from build123d import *

# Parameters (mm, degrees)
F0_W     = 320.8331465721
F0_H     = 70.6209391356
F1_DEPTH = 370
F2_W     = 282.8331465721
F2_H     = 332
F3_DEPTH = 40
F4_W     = 282.8331465721
F4_H     = 332
F5_DEPTH = 40
F6_W     = 360
F6_H     = 145.8556303974
F6_W_2   = 320.8331465721
F6_H_2   = 70.6209391356
F7_DEPTH = 19


with BuildPart() as f1:
    # F0 (on Front) → F1 (new body)
    with BuildSketch(Plane.XZ):
        Rectangle(F0_W, F0_H)
    extrude(amount=F1_DEPTH)

    # F2 (on face) → F3 (join)
    with BuildSketch(Plane.XY.offset(35.3104695678)):
        with Locations((0, -185)):
            Rectangle(F2_W, F2_H)
    extrude(amount=-F3_DEPTH)

    # F4 (on face) → F5 (cut)
    with BuildSketch(Plane.XY.offset(35.3104695678)):
        with Locations((0, -185)):
            Rectangle(F4_W, F4_H)
    extrude(amount=-F5_DEPTH, mode=Mode.SUBTRACT)

    # F6 (on face) → F7 (join)
    with BuildSketch(Plane.XZ.offset(370)):
        Rectangle(F6_W, F6_H)
        Rectangle(F6_W_2, F6_H_2, mode=Mode.SUBTRACT)
        Rectangle(F6_W_2, F6_H_2)
    extrude(amount=F7_DEPTH)


solid = f1.part
For this review, take the finished solid that the model builds, in its own axes (mm). A direction names the side the tool comes from. Round coordinates to 2 decimals unless told otherwise and drop trailing zeros. Write each loop counter-clockwise with the first axis right and the second up, starting at its lowest first coordinate (ties: lowest second). Pieces come first, ordered by that corner, then holes. Notation, with made-up numbers: M 54.5,-1 L 60.5,-1 A30 ccw 60.5,30 Z; hole C 57.25,80 d10. An arc over 180 degrees is marked long. Write item = value, one per line. Start each with the question number.
(1) For faces 5 (the face through (160.417, -182, 0)), 6 (the face through (-160.417, -182, 0)), 7 (the face through (-143, -170, 35.31)), 8 (the face through (141.417, -187, 16)), list the 3-axis set-ups (+Z, -Z, +X, -X, +Y, -Y) from which the entire face can be reached by the end or side of a thin tool; tool diameter is ignored.
(2) For line 1 along Y through (x, z) = (-117, -0.5); line 2 along X through (y, z) = (-256.5, 33.5); line 3 along Z through (x, y) = (-88, -77), list the stretches that pass through material, from the lowest coordinate up.
(3) Clearance check with flat-ended pins moving along their axes: pin 1 Ø3 at (x, y) = (99, -255) entering from +Z; pin 2 Ø20 at (x, z) = (-53, 22) entering from +Y; pin 3 Ø1 at (y, z) = (-238.5, 7.5) entering from +X; pin 4 Ø12 at (y, z) = (-111.5, 20.5) entering from -X. State where each tip first meets the part, or that it passes through.
(4) The part is to be moulded in two halves that separate along Y. For faces 1 (the face through (-2, -19, 16)), 2 (the face through (-3, -379, 72.928)), 3 (the face through (-3, -389, 1)), 4 (the face through (-2, 0, 0)), say which applies: +Y half, -Y half, draft (parallel to the pull), parting line (faces both ways), or undercut.
(5) We need section A-A (z = 7.5). Give the boundary of the cut face in (x, y), then the cut area to 3 significant figures.
(6) We need section B-B (y = -154). Give the boundary of the cut face in (x, z).
(7) We need section C-C (x = -149). Give the boundary of the cut face in (y, z).
(8) We need section D-D (x = 33). Give the boundary of the cut face in (y, z).
Results found:
q1.face_5 = +Z, -Z, +X, +Y
q1.face_6 = +Z, -Z, -X, +Y
q1.face_7 = +Z, +X, -X, +Y
q1.face_8 = +Z
q2.line_1 = -389 to -351, -19 to 0
q2.line_2 = -160.42 to -141.42, 141.42 to 160.42
q2.line_3 = -35.31 to -4.69
q3.pin_1 = -4.69
q3.pin_2 = 0
q3.pin_3 = 160.42
q3.pin_4 = -160.42
q4.face_1 = undercut
q4.face_2 = draft
q4.face_3 = -Y half
q4.face_4 = +Y half
q5.outline = M -180,-389 L 180,-389 L 180,-370 L 160.42,-370 L 160.42,0 L -160.42,0 L -160.42,-370 L -180,-370 Z; hole M -141.42,-351 L 141.42,-351 L 141.42,-19 L -141.42,-19 Z
q5.area = 31,600 mm²
q6.outline = M -160.42,-35.31 L 160.42,-35.31 L 160.42,35.31 L 141.42,35.31 L 141.42,-4.69 L -141.42,-4.69 L -141.42,35.31 L -160.42,35.31 Z
q7.outline = M -389,-72.93 L -370,-72.93 L -370,-35.31 L 0,-35.31 L 0,35.31 L -370,35.31 L -370,72.93 L -389,72.93 Z
q8.outline = M -389,-72.93 L -370,-72.93 L -370,-35.31 L 0,-35.31 L 0,35.31 L -19,35.31 L -19,-4.69 L -351,-4.69 L -351,35.31 L -370,35.31 L -370,72.93 L -389,72.93 Z
